Geometry: final body of the model. Coordinates: model frame, mm. A direction names the side the tool comes from. Give positions to 0.01 mm unless a question says otherwise; leave off trailing zeros. Write each loop counter-clockwise with the first axis right and the second up, starting at its lowest first coordinate (ties: lowest second). Pieces come first, ordered by that corner, then holes.
Q1. Pin query (flat end, axial travel): pin 1 Ø0.6 at (y, z) = (-1, 1) entering from -X; pin 2 Ø1 at (x, y) = (10, 4) entering from -Z. Return the tip coordinate at first contact, or that it passes through.
Q2. Reachability of faces 1 (the flat face through (49, -4.5, 1)), 2 (the flat face through (60, 9, 1)), 3 (the flat face through (-37.5, 0, 1)) from +Z, -Z, +X, -X, +Y, -Y: full face, straight path, thin tool, end or side. Return the list, or none.
Q3. Line query: line 1 (Y direction, x = 42, z = 0.75); line 2 (X direction, y = 0.5, z = 0.55); line 3 (X direction, y = -5.25, z = 1.5). Output: solid intervals per line, ascending.
Q4. Section B-B (z = 1.6). Return the cut outline in (x, y).
Q5. Mould query, pull axis Y, two halves, no side actions, for faces 4 (the flat face through (1, -12.5, 1)), 5 (the flat face through (49, 4.5, 1)), 6 (the flat face through (-60, 8, 1)), 7 (the flat face through (-1, 12.5, 1)). Classes: +Y half, -Y half, draft (parallel to the pull), parting line (faces both ways), or undercut.
Q6. Section A-A (x = 49.5). Return the cut outline in (y, z).
Q7. Section C-C (y = 1.5). Return the cut outline in (x, z), plus the area to 3 significant figures.
Autodesk Fusion 360 part; units mm, degrees
sketch "Sketch1" plane through (0, 0, 0) normal (0, 0, 1) x (1, 0, 0)
  line L0 (-60, 12.5) -> (60, 12.5)
  line L1 (60, 12.5) -> (60, 4.5)
  line L2 (60, 4.5) -> (-60, 4.5)
  line L3 (-60, 4.5) -> (-60, 12.5)
  line L4 (-60, -4.5) -> (60, -4.5)
  line L5 (60, -4.5) -> (60, -12.5)
  line L6 (60, -12.5) -> (-60, -12.5)
  line L7 (-60, -12.5) -> (-60, -4.5)
  line L8 (-37.5, 4.5) -> (37.5, 4.5)
  line L9 (37.5, 4.5) -> (37.5, -4.5)
  line L10 (37.5, -4.5) -> (-37.5, -4.5)
  line L11 (-37.5, -4.5) -> (-37.5, 4.5)
  dimension "d24" = 120
  dimension "d25" = 8
  dimension "d26" = 8
  dimension "d27" = 25
  dimension "d28" = 75
  dimension "d34" = 60
  dimension "d35" = 12.5
  dimension "d38" = 37.5
extrude "Extrude1" add sketch "Sketch1" along normal blind 2
fillet "Fillet1" radius 1 12 edges at (-60, 12.5, 1) (-60, 4.5, 1) (-60, -4.5, 1) (-60, -12.5, 1) (-37.5, 4.5, 1) (-37.5, -4.5, 1) (60, -12.5, 1) (60, -4.5, 1) (37.5, 4.5, 1) (37.5, -4.5, 1) (60, 4.5, 1) (60, 12.5, 1)
equation "d26 = d25"
equation "d34 = d24 / 2"
equation "d35 = d27 / 2"
equation "d38 = d28 / 2"
Computed:
1. pin 1: stops at x = -37.5
1. pin 2: stops at z = 0
2. face 1: +Z, -Z, +X
2. face 2: +Z, -Z, +X, +Y, -Y
2. face 3: +Z, -Z, -X
3. line 1: y = -12.5 to -4.5, 4.5 to 12.5
3. line 2: x = -37.5 to 37.5
3. line 3: x = -59.97 to 59.97
4. outline: (-60, -11.5) arc R1 ccw to (-59, -12.5) - (59, -12.5) arc R1 ccw to (60, -11.5) - (60, -5.5) arc R1 ccw to (59, -4.5) - (38.5, -4.5) arc R1 cw to (37.5, -3.5) - (37.5, 3.5) arc R1 cw to (38.5, 4.5) - (59, 4.5) arc R1 ccw to (60, 5.5) - (60, 11.5) arc R1 ccw to (59, 12.5) - (-59, 12.5) arc R1 ccw to (-60, 11.5) - (-60, 5.5) arc R1 ccw to (-59, 4.5) - (-38.5, 4.5) arc R1 cw to (-37.5, 3.5) - (-37.5, -3.5) arc R1 cw to (-38.5, -4.5) - (-59, -4.5) arc R1 ccw to (-60, -5.5) - close
5. face 4: -Y half
5. face 5: undercut
5. face 6: draft
5. face 7: +Y half
6. outline: (-12.5, 0) - (-4.5, 0) - (-4.5, 2) - (-12.5, 2) - close; (4.5, 0) - (12.5, 0) - (12.5, 2) - (4.5, 2) - close
7. outline: (-37.5, 0) - (37.5, 0) - (37.5, 2) - (-37.5, 2) - close
7. area: 150 mm2
